Can you work these out from the model? Positions are in its coordinate system, mm. Face numbers are marked on the shaded views. A direction names the side the tool comes from. Round coordinates to 2 decimals unless told otherwise and drop trailing zeros. Order: outer loops, then holes, each group sorted by start corner. A loop starts at its lowest first (then second) coordinate and runs counter-clockwise, first axis right, second up. Notation, with made-up numbers: (-14, 69.25) -> (28, 69.25) arc R7 ccw to (28, 76.25) -> close; hole circle Ø1 at (-33.75, 32.5). An arc over 180 degrees is marked (long way). Use a Markdown table: item, result. Add a question column.
Q1. If we section it at A-A on y = 8.5: List the corners of the cut face in (x, z) for me, plus the area to 3 significant figures.
Q2. We'd pull the mould along Y, two halves only. Please class the marked faces 1, 2 and 3: +Y half, -Y half, draft (parallel to the pull), parting line (faces both ways), or undercut.
Q3. I need wall thicknesses on line 1 along Y through (x, z) = (2.75, 0); line 2 along Y through (x, z) = (-4.05, -26.6); line 3 along Y through (x, z) = (-1.7, -18.6). Which ranges of each line are inside material? Lowest first, please. Write a range as [from, to].
Q4. If we section it at B-B on z = -18.6: List the corners of the cut face in (x, y) for me, plus the area to 3 significant figures.
Q5. If we section it at D-D on z = -1: List the corners of the cut face in (x, y) for me.
Q6. If we section it at C-C on x = -2.5: List the corners of the cut face in (y, z) for me, plus the area to 3 significant figures.
Q7. For the marked faces 4, 5 and 6, which set-ups out of +Z, -Z, +X, -X, +Y, -Y let a thin tool reach every point of the face, with its end or its side?
Q8. I'm going to push flat-ended pins straight in: pin 1 Ø9.5 at (y, z) = (12, -10.6) entering from +X; pin 2 Ø4 at (x, y) = (-1, 23) entering from +Z; pin 3 Ø3.5 at (y, z) = (20, -18.6) entering from -X. Where does each tip first touch, or does it pass through?
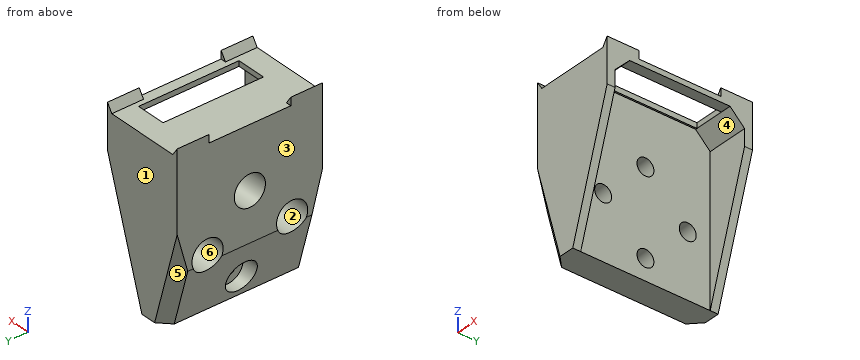
Autodesk Inventor part; units mm, degrees
ref_plane "Work Plane1" through (-3, 0, 4) normal (1, 0, 0) x (0, 0, -1)
ref_plane "Work Plane2" through (0, 12, 0) normal (0, -1, 0) x (1, 0, 0)
ref_plane "YZ Plane" through (0, 0, 0) normal (1, 0, 0) x (0, 1, 0)
sketch "Sketch1" plane through (0, 0, 0) normal (0, 1, 0) x (-1, 0, 0)
  line L0 (0, 0) -> (0, -30.6)
  line L1 (0, -30.6) -> (5, -30.6)
  line L2 (0, 0) -> (13.774, 0)
  line L3 (13.774, 0) -> (5, -30.6)
  line L4 (13.774, 0) -> (13.774, 4)
  line L5 (0, 0) -> (0, 9.5471)
  line L6 (13.774, 4) -> (-10.8744, 4)
  point P0 (0, 4)
  dimension "d0" = 30.6
  dimension "d1" = 5
  dimension "d2" = 13.774
  dimension "d3" = 4
extrude "Extrusion1" add sketch "Sketch1" along normal blind 24
sketch "Sketch2" plane through (0, 0, 4) normal (1, 0, 0) x (0, 0, -1)
  line L0 (34.6, 0) -> (34.6, 24)
  line L1 (34.6, 12) -> (30.6, 12)
  line L2 (30.6, 12) -> (14.6, 12)
  line L3 (22.6, 12) -> (22.6, 20)
  line L4 (22.6, 12) -> (22.6, 4)
  circle A0 centre (22.6, 20) radius 1.6
  circle A1 centre (14.6, 12) radius 1.6
  circle A2 centre (22.6, 4) radius 1.6
  circle A3 centre (30.6, 12) radius 1.6
  point P0 (4, 0)
  dimension "d6" = 4
  dimension "d7" = 16
  dimension "d8" = 8
  dimension "d9" = 8
  dimension "d10" = 3.2
  dimension "d11" = 3.2
  dimension "d12" = 3.2
  dimension "d13" = 3.2
extrude "Extrusion2" cut sketch "Sketch2" against normal blind 24
ref_plane "Work Plane1" through (-3, 0, 4) normal (1, 0, 0) x (0, 0, -1)
sketch "Sketch3" plane through (-3, 0, 4) normal (1, 0, 0) x (0, 0, -1)
  circle A0 centre (22.6, 20) radius 1.6
  circle A1 centre (22.6, 20) radius 2.95
  circle A2 centre (14.6, 12) radius 1.6
  circle A3 centre (14.6, 12) radius 2.95
  circle A4 centre (22.6, 4) radius 1.6
  circle A5 centre (22.6, 4) radius 2.95
  circle A6 centre (30.6, 12) radius 1.6
  circle A7 centre (30.6, 12) radius 2.95
  point P0 (4, 0)
  dimension "d17" = 5.9
  dimension "d18" = 5.9
  dimension "d19" = 5.9
  dimension "d20" = 5.9
extrude "Extrusion3" cut sketch "Sketch3" against normal blind 24 contours A0 | A1 | A2 | A3 | A4 | A5 | A6 | A7
sketch "Sketch5" plane through (0, 0, 4) normal (1, 0, 0) x (0, 0, -1)
  line L0 (4, 0) -> (0, 0)
  line L1 (34.6, 24) -> (4, 24)
  line L2 (0, 0) -> (4, 0)
  line L3 (4, 0) -> (4, 24)
  line L4 (4, 24) -> (0, 24)
  line L5 (0, 24) -> (0, 0)
  line L6 (4, 0) -> (4, 24)
  line L7 (4, 24) -> (6.5, 24)
  line L8 (6.5, 24) -> (6.5, 21.5)
  line L9 (6.5, 21.5) -> (4, 21.5)
  line L10 (4, 21.5) -> (4, 24)
  line L11 (4, 0) -> (6.5, 0)
  line L12 (6.5, 0) -> (6.5, 2.5)
  line L13 (6.5, 2.5) -> (4, 2.5)
  line L14 (4, 2.5) -> (4, 0)
  line L15 (4, 2.5) -> (6.5, 0)
  line L16 (4, 21.5) -> (6.5, 24)
  dimension "d40" = 4
  dimension "d41" = 24
  dimension "d44" = 2.5
  dimension "d45" = 2.5
  dimension "d46" = 2.5
  dimension "d47" = 2.5
extrude "Extrusion6" add sketch "Sketch5" along normal blind 8.9 contours L0 L5 L4 L3 | L3 L15 L11 | L3 L1 L16
sketch "Sketch7" plane through (0, 2.5, 0) normal (0, 0, -1) x (-1, 0, 0)
  line L0 (0, 0) -> (-8.9, 0)
  line L1 (0, 19) -> (-8.9, 19)
  line L2 (0, 0) -> (-5.5, 0)
  line L3 (-5.5, 0) -> (-5.5, 19)
  line L4 (-5.5, 19) -> (0, 19)
  line L5 (0, 19) -> (0, 0)
  line L6 (0, 21.5) -> (0, 19)
  line L7 (0, 19) -> (-0.3, 19)
  line L8 (-0.3, 19) -> (-0.3, 0)
  line L9 (-0.3, 0) -> (0, 0)
  line L10 (0, 0) -> (0, 19)
  point P0 (0, -2.5)
  dimension "d55" = 5.5
  dimension "d56" = 0.3
extrude "Extrusion8" cut sketch "Sketch7" against normal blind 30 contours L0 L3 L1 L8
sketch "Sketch9" plane through (-13.774, 0, 0) normal (-1, 0, 0) x (0, 0, 1)
  line L0 (-2.5, 24) -> (-30.6, 24)
  line L1 (4, 0) -> (-30.6, 0)
  line L2 (-30.6, 0) -> (-30.6, 24)
  line L3 (-30.6, 24) -> (4, 24)
  line L4 (4, 24) -> (4, 0)
  point P0 (0, 0)
extrude "Extrusion10" cut sketch "Sketch9" against normal blind 5.674
sketch "Sketch10" plane through (8.9, 0, 4) normal (1, 0, 0) x (0, 0, -1)
  line L0 (6.5, 24) -> (0, 24)
  line L1 (0, 24) -> (0, 24.25)
  line L2 (0, 24.25) -> (8.0681, 24.25)
  line L3 (4, 21.5) -> (6.5, 24)
  line L4 (4, 21.5) -> (7.5355, 25.0355)
  line L5 (4, 21.5) -> (9, 21.5) construction
  line L6 (0, 24) -> (0, 0)
  line L7 (6.5, 24) -> (0, 24)
  line L8 (4, 21.5) -> (4, 2.5)
  line L9 (4, 12) -> (-3.3365, 12)
  line L10 (6.5, 0) -> (0, 0)
  line L11 (0, 0) -> (0, -0.25)
  line L12 (0, -0.25) -> (8.0681, -0.25)
  line L13 (4, 2.5) -> (6.5, 0)
  line L14 (4, 2.5) -> (7.5355, -1.0355)
  line L15 (4, 2.5) -> (9, 2.5) construction
  line L16 (6.5, 0) -> (0, 0)
  point P0 (4, 0)
  point P1 (6.75, -0.25)
  point P2 (6.75, 24.25)
  dimension "d65" = 0.25
  dimension "d66" = 5
  dimension "d67" = 45
extrude "Extrusion11" add sketch "Sketch10" against normal blind 8.9 contours L0 L1 L2 L4 | L10 L14 L12 L11
ref_plane "Work Plane2" through (0, 12, 0) normal (0, -1, 0) x (1, 0, 0)
sketch "Sketch12" plane through (8.9, -0.25, -2.75) normal (0, -1, 0) x (1, 0, 0)
  line L0 (0, 0) -> (0, 2.75)
  line L1 (0, 0) -> (-8.9, 0)
  line L2 (-8.9, 0) -> (-8.9, 6.75)
  line L3 (-8.9, 6.75) -> (0, 6.75)
  line L4 (0, 6.75) -> (0, 0)
  point P0 (-8.9, 2.75)
extrude "Extrusion12" add sketch "Sketch12" along normal blind 1.5
sketch "Sketch13" plane through (0, 0, 0) normal (0, -1, 0) x (1, 0, 0)
  line L0 (0, -30.6) -> (-5, -30.6)
  line L1 (0, -2.5) -> (0, 4)
  line L2 (-5, -30.6) -> (0, -30.6)
  line L3 (0, -30.6) -> (0, 4)
  line L4 (0, 4) -> (-5, 4)
  line L5 (-5, 4) -> (-5, -30.6)
  line L6 (-8.1, -19.7885) -> (-5, -19.7885)
  line L7 (-5, -19.7885) -> (-5, 4)
  line L8 (-5, 4) -> (-8.1, 4)
  line L9 (-8.1, 4) -> (-8.1, -19.7885)
  line L10 (-5, -30.6) -> (-8.1, -19.7885)
  line L11 (-5, -30.6) -> (-8.1, -19.7885)
  point P0 (0, 0)
extrude "Extrusion13" add sketch "Sketch13" along normal blind 1.75
sketch "Sketch14" plane through (8.9, -1.75, -2.75) normal (0, -1, 0) x (1, 0, 0)
  line L0 (-8.9, -27.85) -> (-8.9, 0)
  line L1 (0, 0) -> (0, 2.75)
  line L2 (-8.9, -27.85) -> (0, 0)
  line L3 (-8.9, -27.85) -> (0, -27.85)
  line L4 (0, -27.85) -> (0, 0)
  line L5 (0, 0) -> (-8.9, 0)
  line L6 (-8.9, 0) -> (-8.9, -27.85)
  point P0 (-8.9, 2.75)
  point P1 (-8.9, 0)
extrude "Extrusion14" add sketch "Sketch14" against normal blind 1.5 contours L0 L5 L2
mirror "Mirror1" about plane through (0, 12, 0) normal (0, -1, 0) of "Extrusion12", "Extrusion13", "Extrusion14"
sketch "Sketch15" plane through (8.9, 0, 4) normal (1, 0, 0) x (0, 0, -1)
  line L0 (22.1903, 31.1847) -> (-2.991, 31.1847)
  line L1 (-2.991, 31.1847) -> (-2.991, -5.1617)
  line L2 (-2.991, -5.1617) -> (22.1903, -5.1617)
  line L3 (22.1903, -5.1617) -> (22.1903, 31.1847)
  point P0 (4, 0)
extrude "Extrusion17" cut sketch "Sketch15" against normal blind 1
sketch "Sketch16" plane through (-8.1, -1.75, 4) normal (0, 0, 1) x (1, 0, 0)
  line L0 (23.1984, -4.3461) -> (-2.2485, -4.3461)
  line L1 (-2.2485, -4.3461) -> (-2.2485, 32.2961)
  line L2 (-2.2485, 32.2961) -> (23.1984, 32.2961)
  line L3 (23.1984, 32.2961) -> (23.1984, -4.3461)
  point P0 (8.1, 1.75)
extrude "Extrusion18" cut sketch "Sketch16" against normal blind 3
sketch "Sketch17" plane through (5.5, 2.5, 0) normal (0, 0, -1) x (-1, 0, 0)
  line L0 (5.2, 0) -> (0, 0)
  line L1 (-2.4, 19) -> (-2.4, 0)
  line L2 (0, 0) -> (-2.4, 0)
  line L3 (-2.4, 0) -> (-2.4, 19)
  line L4 (-2.4, 19) -> (0, 19)
  line L5 (0, 19) -> (0, 0)
  point P0 (5.5, -2.5)
extrude "Extrusion19" cut sketch "Sketch17" against normal blind 3
sketch "Sketch18" plane through (8.9, -1.75, -2.75) normal (0, -1, 0) x (1, 0, 0)
  line L0 (-8.6, 3.75) -> (-1, 3.75)
  line L1 (-1, 3.75) -> (-3, 3.75)
  line L2 (-1, 5.75) -> (-1, 3.75)
  line L3 (-1, 3.75) -> (-2, 3.75)
  line L4 (-2, 3.75) -> (-2, 5.25)
  line L5 (-2, 5.25) -> (-1, 5.25)
  line L6 (-1, 5.25) -> (-1, 3.75)
  line L7 (-1, 5.25) -> (-2, 3.75)
  point P0 (-8.9, 2.75)
  point P1 (-2, 3.75)
  dimension "d97" = 1
  dimension "d98" = 1.5
extrude "Extrusion20" add sketch "Sketch18" against normal blind 27.5 contours L7 L2 L0
sketch "Sketch19" plane through (7.9, 2.5, 1) normal (0, 0, -1) x (-1, 0, 0)
  line L0 (7.6, 19) -> (0, 19)
  line L1 (7.6, 0) -> (0, 0)
  line L2 (0, 19) -> (2, 19)
  line L3 (2, 19) -> (2, 0)
  line L4 (2, 0) -> (0, 0)
  line L5 (0, 0) -> (0, 19)
  point P0 (7.9, -2.5)
  dimension "d101" = 2
extrude "Extrusion21" add sketch "Sketch19" along normal blind 1
sketch "Sketch20" plane through (8.9, -1.75, -2.75) normal (0, -1, 0) x (1, 0, 0)
  line L0 (-1, 5.25) -> (-1, -3.1292)
  line L1 (-1, 5.25) -> (-17, 5.25)
  line L2 (-17, 5.25) -> (-17, 0.25)
  line L3 (-17, 5.25) -> (-16, 5.25)
  line L4 (-16, 5.25) -> (-16, 3.75)
  line L5 (-16, 3.75) -> (-17, 3.75)
  line L6 (-17, 3.75) -> (-17, 5.25)
  line L7 (-17, 5.25) -> (-16, 3.75)
  point P0 (-8.9, 2.75)
  dimension "d107" = 16
  dimension "d108" = 5
  dimension "d109" = 1
  dimension "d110" = 1.5
extrude "Extrusion22" add sketch "Sketch20" against normal blind 27.5 contours L7 L5 L2
sketch "Sketch21" plane through (7.9, 0, 4) normal (1, 0, 0) x (0, 0, -1)
  line L0 (1.5, -1.75) -> (1.5, 25.75)
  line L1 (1.5, -1.75) -> (1.5, 4.25)
  line L2 (1.5, 25.75) -> (9.8792, 25.75)
  line L3 (1.5, 25.75) -> (1.5, 19.75)
  line L4 (1.5, 19.75) -> (3, 19.75)
  line L5 (3, 21.5) -> (3, 2.5)
  line L6 (1.5, 19.75) -> (1.5, 4.25)
  line L7 (1.5, 4.25) -> (3, 4.25)
  line L8 (3, 4.25) -> (3, 19.75)
  point P0 (4, 0)
  dimension "d116" = 6
  dimension "d117" = 6
extrude "Extrusion23" cut sketch "Sketch21" against normal blind 60
chamfer "Chamfer9" distance 2 angle 45 2 edges at (-6.55, 25.75, -25.1943) (-6.55, -1.75, -25.1943)
properties part number "finger_v1"
Answer below:
| question | item | result |
|---|---|---|
| 1 | outline | (-8.1, -19.79) -> (-5, -30.6) -> (0, -30.6) -> (0, 0) -> (0.3, 0) -> (0.3, 1) -> (-8.1, 1) -> close; (5.9, 0) -> (7.9, 0) -> (7.9, 1) -> (5.9, 1) -> close |
| 1 | area | 242 mm² |
| 2 | face 1 | +Y half |
| 2 | face 2 | undercut |
| 2 | face 3 | draft |
| 3 | line 1 | [-1.75, 2.5], [21.5, 25.75] |
| 3 | line 2 | [-1.75, 9.05], [14.95, 25.75] |
| 3 | line 3 | [-1.75, 2.4], [5.6, 18.4], [21.6, 25.75] |
| 4 | outline | (-8.1, -0.08) -> (-6.36, -1.75) -> (3.83, -1.75) -> (3.83, -0.25) -> (0, -0.25) -> (0, 2.4) -> (-3, 2.4) -> (-3, 1.05) -> (-8.1, 1.05) -> close; (-8.1, 6.95) -> (-3, 6.95) -> (-3, 5.6) -> (0, 5.6) -> (0, 18.4) -> (-3, 18.4) -> (-3, 17.05) -> (-8.1, 17.05) -> close; (-8.1, 22.95) -> (-3, 22.95) -> (-3, 21.6) -> (0, 21.6) -> (0, 24.25) -> (3.83, 24.25) -> (3.83, 25.75) -> (-6.36, 25.75) -> (-8.1, 24.08) -> close |
| 4 | area | 152 mm² |
| 5 | outline | (-8.1, -1.75) -> (7.9, -1.75) -> (7.9, 1.5) -> (0, 1.5) -> (0, 22.5) -> (7.9, 22.5) -> (7.9, 25.75) -> (-8.1, 25.75) -> close |
| 6 | outline | (-1.75, -30.6) -> (25.75, -30.6) -> (25.75, 1) -> (-1.75, 1) -> close; hole circle Ø3.2 at (4, -18.6); hole circle Ø3.2 at (12, -26.6); hole circle Ø3.2 at (12, -10.6); hole circle Ø3.2 at (20, -18.6) |
| 6 | area | 837 mm² |
| 7 | face 4 | -Z, +X |
| 7 | face 5 | -Z, -X, +Y |
| 7 | face 6 | -X |
| 8 | pin 1 | x = 0 |
| 8 | pin 2 | z = 1 |
| 8 | pin 3 | x = -3 |
